```python
from build123d import *


with BuildPart() as f1:
    # F0 (on Front) → F1 (revolve)
    with BuildSketch(Plane.XZ):
        with BuildLine():
            Line((-9.0625, 0), (-3.875, 0))
            ThreePointArc((-3.875, 0), (-3.256282, 0.256282), (-3, 0.875))
            Line((-3, 0.875), (-3, 7.75))
            Line((-3, 7.75), (-3.875, 7.75))
            Line((-3.875, 7.75), (-3.875, 1.419101))
            ThreePointArc((-3.875, 1.419101), (-4.003141, 1.109741), (-4.3125, 0.981601))
            Line((-4.3125, 0.981601), (-9.0625, 0.981601))
            ThreePointArc((-9.0625, 0.981601), (-9.371859, 0.85346), (-9.5, 0.544101))
            Line((-9.5, 0.544101), (-9.5, 0.4375))
            ThreePointArc((-9.5, 0.4375), (-9.371859, 0.128141), (-9.0625, 0))
        make_face()
    revolve(axis=Axis((0, 0, 3.875), (0, 0, 1)))


solid = f1.part
```
Model file for the job. Use its own axes, mm. A direction names the side the tool comes from. Give positions to 0.01 mm unless a question says otherwise; leave off trailing zeros. Loops run counter-clockwise (first coordinate to the right, second up) from the corner with the lowest first, then second, coordinate; pieces in that order, holes last. Notation, with made-up numbers: (-4.5, 62) -> (38.5, 62) arc R20 ccw to (38.5, 87) -> close; hole circle Ø2 at (46, 12.25). An arc over 180 degrees is marked (long way). Use CSV: the item, a comma, the result in double quotes. Start each with the question number.
1) Tool access for faces 1 (the cylindrical face through (3, 0, 4)), 2 (the cylindrical face through (0.504, -3.842, 4.54)): list every direction of +Z, -Z, +X, -X, +Y, -Y with a clear straight run to the whole face (end or side of a thin tool).
2) Flat gauge pin, fed straight in: pin 1 Ø3 at (x, z) = (-0.5, 6.5) entering from +Y (3 decimals). Where does the tip first touch, or does it go through?
3) Wall check: line 1 (X direction, y = 0, z = 4.75) (3 decimals); line 2 (Z direction, x = 0.25, y = 4.5). Give the ranges that are in metal, low to high.
4) Slice it at C-C on z = 3.5. Give the cut face in (x, y) (3 decimals).
Computed values:
1,face 1,"+Z, -Z"
1,face 2,"+Z"
2,pin 1,"stops at y = 3.875"
3,line 1,"x = -3.875 to -3, 3 to 3.875"
3,line 2,"z = 0 to 0.98"
4,outline,"circle Ø7.75 at (0, 0); hole circle Ø6 at (0, 0)"
